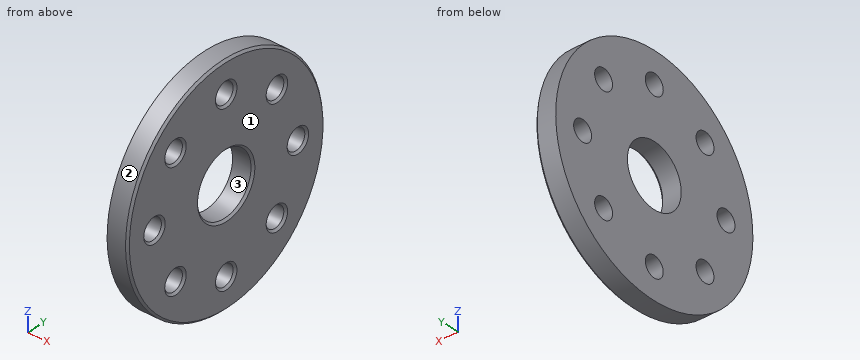
from build123d import *

# Parameters (mm, degrees)
SKETCH2_W          = 2
SKETCH2_H          = 8
SKETCH3_R          = 1
CUT_EXTRUDE1_DEPTH = 16.684387141
CIRPATTERN1_COUNT  = 8
CHAMFER1_SIZE      = 0.2


with BuildPart() as part:
    # Sketch2 → Revolve1 (revolve)
    with BuildSketch(Plane.XY, mode=Mode.PRIVATE) as revolve1_sk:
        with Locations((0, 7)):
            Rectangle(SKETCH2_W, SKETCH2_H)
    revolve(revolve1_sk.sketch.rotate(Axis((0, 0, 0), (1, 0, 0)), 90), axis=Axis((0, 0, 0), (1, 0, 0)))

    # Sketch3 → Cut-Extrude1 (cut, through all)
    with BuildSketch(Plane.ZY.offset(1)):
        with Locations((0, 8)):
            Circle(SKETCH3_R)
    cut_extrude1 = extrude(amount=-CUT_EXTRUDE1_DEPTH, mode=Mode.SUBTRACT)

    # CirPattern1: Cut-Extrude1 ×8 about axis
    cirpattern1_axis = Axis((0, 0, 0), (1, 0, 0))
    for i in range(1, CIRPATTERN1_COUNT):
        add(cut_extrude1.rotate(cirpattern1_axis, i * 360 / CIRPATTERN1_COUNT), mode=Mode.SUBTRACT)

    # Chamfer1
    chamfer1_edges = [part.edges().sort_by_distance(p)[0] for p in [
        (1, 8, -1),
        (1, 4.949747468, -6.363961031),
        (1, -1, -8),
        (1, -6.363961031, -4.949747468),
        (1, -8, 1),
        (1, -4.949747468, 6.363961031),
        (1, 1, 8),
        (1, 0, -3),
        (1, 0, -11),
        (1, 6.363961031, 4.949747468),
    ]]
    chamfer(chamfer1_edges, length=CHAMFER1_SIZE)


solid = part.part
The model under review builds one solid part; all positions refer to its coordinate system, in mm. Face numbers are marked on the shaded views. Round coordinates to 2 decimals unless told otherwise and drop trailing zeros. Write each loop counter-clockwise with the first axis right and the second up, starting at its lowest first coordinate (ties: lowest second). Pieces come first, ordered by that corner, then holes. Notation, with made-up numbers: (-24, -8.5) - (35, -8.5) arc R20 ccw to (35, 25.5) - close; hole circle Ø10 at (-36.75, 58.25). An arc over 180 degrees is marked (long way). One line per item, written item: value. Start each with the question number.
1. To check wall thickness, follow L1, parallel to Z at x = -0.9, y = 4.75; L2, parallel to Z at x = 0.15, y = -5.5. State the ranges of each line that lie inside material, in increasing order. Write a range as from..to.
2. Consider section A-A on z = 0. Write out the cut boundary in (x, y).
3. Consider section B-B on x = 0.5. State how many separate pieces and enclosed holes the cut face has, and give its area (3 significant figures).
4. The part is to be moulded in two halves that separate along Z. For the marked faces 1, 2 and 3, say which applies: released by +Z, released by -Z, zero draft, split by the parting line, or undercut.
Checks:
1. L1: z = -9.92..-6.08, -5.24..5.24, 6.08..9.92
1. L2: z = -9.53..-6.64, -4.67..4.67, 6.64..9.53
2. outline: (-1, -11) - (0.8, -11) - (1, -10.8) - (1, -9.2) - (0.8, -9) - (-1, -9) - close; (-1, -7) - (0.8, -7) - (1, -6.8) - (1, -3.2) - (0.8, -3) - (-1, -3) - close; (-1, 3) - (0.8, 3) - (1, 3.2) - (1, 6.8) - (0.8, 7) - (-1, 7) - close; (-1, 9) - (0.8, 9) - (1, 9.2) - (1, 10.8) - (0.8, 11) - (-1, 11) - close
3. separate pieces: 1
3. enclosed holes: 9
3. area: 327 mm^2
4. face 1: zero draft
4. face 2: split by the parting line
4. face 3: undercut
